from build123d import *

# Parameters (mm, degrees)
EXTRUDE_1_DEPTH     = 35
SKETCH_2_R          = 1.5
CUT_EXTRUDE_1_DEPTH = 5
SKETCH_3_R          = 1.5
EXTRUDE_2_DEPTH     = 5


with BuildPart() as part:
    # 草图1 → 凸台-拉伸1 (new body)
    with BuildSketch(Plane(origin=(0, 0, 0), x_dir=(1, 0, 0), z_dir=(0, 1, 0))):
        Polygon((2.528327266, -1.393159922), (2.470675517, 1.49301568), (-0.057651749, 2.886175603), (-2.528327266, 1.393159922), (-2.470675517, -1.49301568), (0.057651749, -2.886175603), align=None)
    extrude(amount=EXTRUDE_1_DEPTH)

    # 草图2 → 切除-拉伸1 (cut)
    with BuildSketch(Plane.XZ):
        with Locations(Location((0, 0, 0), (0, 0, 270))):
            Circle(SKETCH_2_R)
    extrude(amount=-CUT_EXTRUDE_1_DEPTH, mode=Mode.SUBTRACT)

    # 草图3 → 凸台-拉伸2 (add)
    with BuildSketch(Plane(origin=(0, 35, 0), x_dir=(1, 0, 0), z_dir=(0, 1, 0))):
        with Locations(Location((0, 0, 0), (0, 0, 90))):
            Circle(SKETCH_3_R)
    extrude(amount=EXTRUDE_2_DEPTH)


solid = part.part
Could you check a few things on this model? Use its own coordinates, in mm. A direction names the side the tool comes from. Coordinates: 2 decimals unless noted, no trailing zeros. Loops run counter-clockwise (first coordinate to the right, second up) from the corner with the lowest first, then second, coordinate; pieces in that order, holes last.
1. We'd pull the mould along X, two halves only. Please class faces 3 (the face through (0.45, 2.46, -1.43)), 4 (the face through (-1.2, 35, 1.2)), 5 (the face through (-0.45, 37.47, -1.43)), 6 (the face through (-1.22, 17.26, 2.18)): released by +X, released by -X, zero draft, split by the parting line, or undercut.
2. For faces 1 (the face through (0, 5, 0)), 2 (the face through (1.276, 17.255, 2.15)), which set-ups out of +Z, -Z, +X, -X, +Y, -Y let a thin tool reach every point of the face, with its end or its side?
3. Imagine slicing it at B-B (x = 0.55). Please give me the cut outline in (y, z), and give its area (3 significant figures).
4. I need wall thicknesses on L1, parallel to Y at x = -0.45, z = 1.1; L2, parallel to X at y = 1.55, z = 0; L3, parallel to Y at x = 1.25, z = 1.05. Which ranges of each line are inside material? Lowest first, please.
5. For P1, Ø2, axis at y = 34.5, z = 0, coming from the -X side, with a flat end and sliding along its axis, tell me the tip position at first contact or that it passes through.
6. Imagine slicing it at A-A (z = 0.85). Please give me the cut outline in (x, y), and give its area (3 significant figures).
7. Imagine slicing it at D-D (x = -1.95). Please give me the cut outline in (y, z).
8. Imagine slicing it at C-C (y = 19.5). Please give me the cut outline in (x, z).
Computed values:
1. face 3: undercut
1. face 4: zero draft
1. face 5: split by the parting line
1. face 6: released by -X
2. face 1: -Y
2. face 2: +Z, +X, +Y, -Y
3. outline: (0, -2.55) - (35, -2.55) - (35, -1.4) - (40, -1.4) - (40, 1.4) - (35, 1.4) - (35, 2.59) - (0, 2.59) - (0, 1.4) - (5, 1.4) - (5, -1.4) - (0, -1.4) - close
3. area: 180 mm2
4. L1: y = 5 to 40
4. L2: x = -2.5 to -1.5, 1.5 to 2.5
4. L3: y = 0 to 35
5. P1: stops at x = -2.52
6. outline: (-2.48, 0) - (-1.24, 0) - (-1.24, 5) - (1.24, 5) - (1.24, 0) - (2.52, 0) - (2.52, 35) - (1.24, 35) - (1.24, 40) - (-1.24, 40) - (-1.24, 35) - (-2.48, 35) - close
6. area: 175 mm2
7. outline: (0, -1.74) - (35, -1.74) - (35, 1.78) - (0, 1.78) - close
8. outline: (-2.53, -1.39) - (-0.06, -2.89) - (2.47, -1.49) - (2.53, 1.39) - (0.06, 2.89) - (-2.47, 1.49) - close
